The model under review builds one solid part; all positions refer to its coordinate system, in mm. Coordinates: 2 decimals unless noted, no trailing zeros. Write each loop counter-clockwise with the first axis right and the second up, starting at its lowest first coordinate (ties: lowest second). Pieces come first, ordered by that corner, then holes. Notation, with made-up numbers: (81.25, 13) - (128.25, 13) arc R34 cw to (128.25, 49) - close; hole circle Ø1 at (63.5, -38). An arc over 180 degrees is marked (long way). Put each result on its own line as item: value. Start each with the question number.
Item 1: For pin 1 (4.5 mm diameter, centred on x = 15.5, z = 50, fed in from -Y), flat-tipped, find the tip position at first contact; note if it passes through.
Item 2: Consider section A-A on x = -4.5. Give the boundary of the cut face in (y, z), then the cut area to 3 significant figures.
Item 3: To check wall thickness, follow L1, parallel to Z at x = 12.5, y = -35.15; L2, parallel to X at y = -33.75, z = 70; L3, parallel to Z at x = -14.5, y = -34.25. State the ranges of each line that lie inside material, in increasing order. Write a range as [from, to].
Item 4: Consider section D-D on x = 12.5. Give the boundary of the cut face in (y, z).
Item 5: Consider section C-C on z = 70. Give the boundary of the cut face in (x, y), then the cut area to 3 significant figures.
Item 6: Consider section B-B on z = 4.5. Give the boundary of the cut face in (x, y), then the cut area to 3 significant figures.
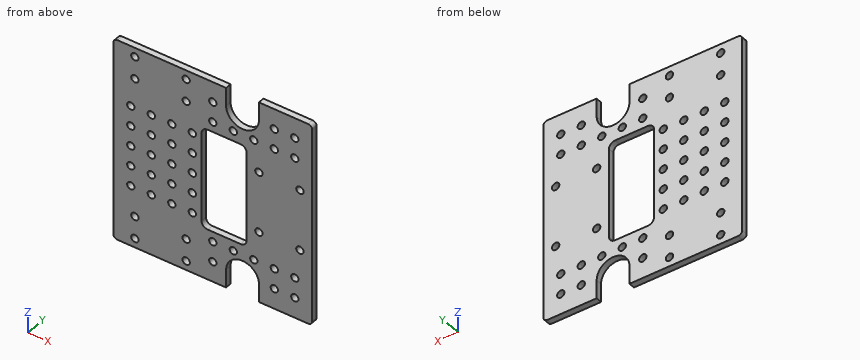
```python
from build123d import *

# Parameters (mm, degrees)
CYLINDER038_R            = 1.8
CYLINDER038_DEPTH        = 100
ARRAY001_X_COUNT         = 2
ARRAY001_X_PITCH         = 25
ARRAY001_Y_COUNT         = 2
ARRAY001_Y_PITCH         = 11
ARRAY001_PLACEMENT_ANGLE = 90
ARRAY002_Z_COUNT         = 2
ARRAY002_Z_PITCH         = 80
CYLINDER011003_R         = 1.8
CYLINDER011003_DEPTH     = 10
ARRAY005_X_COUNT         = 2
ARRAY005_X_PITCH         = 30
ARRAY005_Y_COUNT         = 2
ARRAY005_Y_PITCH         = 20
ARRAY005_PITCH_ANGLE     = 90
ARRAY005_PLACEMENT_ANGLE = -90
BOX002_W                 = 22
BOX002_H                 = 10
BOX002_DEPTH             = 50
FILLET002_R              = 3
BOX003_W                 = 16
BOX003_H                 = 200
BOX003_DEPTH             = 50
CYLINDER_R               = 8
CYLINDER_DEPTH           = 200
SKETCH_W                 = 42.117567
SKETCH_H                 = 23.738708
SKETCH_W_2               = 40.471139
SKETCH_H_2               = 27.047569
SKETCH_W_3               = 29.381024
SKETCH_H_3               = 46.19655
EXTRUDE_DEPTH            = 50
CYLINDER011002_R         = 1.8
CYLINDER011002_DEPTH     = 100
ARRAY004_X_COUNT         = 9
ARRAY004_X_PITCH         = 10
ARRAY004_Z_COUNT         = 9
ARRAY004_Z_PITCH         = 10
BOX_W                    = 97
BOX_H                    = 3
BOX_DEPTH                = 100
FILLET_R                 = 2


with BuildPart() as bolt_hole_array_pair:
    # Cylinder038 → Cylinder038 (new body)
    with BuildSketch(Plane.XY.offset(-50)):
        Circle(CYLINDER038_R)
    extrude(amount=CYLINDER038_DEPTH)

    # Array001 X: bolt hole array pair ×2


with BuildPart() as bolt_hole_array_pair_1:
    add(bolt_hole_array_pair.part)
    with Locations(*[(i * ARRAY001_X_PITCH, 0, 0) for i in range(1, ARRAY001_X_COUNT)]):
        add(bolt_hole_array_pair.part)

    # Array001 Y: bolt hole array pair ×2


with BuildPart() as bolt_hole_array_pair_2:
    add(bolt_hole_array_pair_1.part)
    with Locations(*[(0, i * ARRAY001_Y_PITCH, 0) for i in range(1, ARRAY001_Y_COUNT)]):
        add(bolt_hole_array_pair_1.part)


with BuildPart() as bolt_hole_array_pair_3:
    # Array001 placement: moved
    add(bolt_hole_array_pair_2.part.moved(Location((-12.5, 0, 4.5))).rotate(Axis((-12.5, 0, 4.5), (1, 0, 0)), ARRAY001_PLACEMENT_ANGLE))

    # Array002 Z: bolt hole array pair ×2


with BuildPart() as bolt_hole_array_pair_4:
    add(bolt_hole_array_pair_3.part)
    with Locations(*[(0, 0, i * ARRAY002_Z_PITCH) for i in range(1, ARRAY002_Z_COUNT)]):
        add(bolt_hole_array_pair_3.part)


with BuildPart() as stepper_mount_hole_array:
    # Cylinder011003 → Cylinder011003 (new body)
    with BuildSketch(Plane.XY):
        Circle(CYLINDER011003_R)
    extrude(amount=CYLINDER011003_DEPTH)

    # Array005 X: stepper mount hole array ×2


with BuildPart() as stepper_mount_hole_array_1:
    add(stepper_mount_hole_array.part)
    with Locations(*[(i * ARRAY005_X_PITCH, 0, 0) for i in range(1, ARRAY005_X_COUNT)]):
        add(stepper_mount_hole_array.part)

    # Array005 Y: stepper mount hole array ×2


with BuildPart() as stepper_mount_hole_array_2:
    add(stepper_mount_hole_array_1.part)
    with Locations(*[(0, i * ARRAY005_Y_PITCH, 0) for i in range(1, ARRAY005_Y_COUNT)]):
        add(stepper_mount_hole_array_1.part)


with BuildPart() as stepper_mount_hole_array_3:
    # Array005 pitch: moved
    add(stepper_mount_hole_array_2.part.rotate(Axis((0, 0, 0), (0, 1, 0)), ARRAY005_PITCH_ANGLE))


with BuildPart() as stepper_mount_hole_array_4:
    # Array005 placement: moved
    add(stepper_mount_hole_array_3.part.moved(Location((48, -31, 65))).rotate(Axis((48, -31, 65), (0, 0, 1)), ARRAY005_PLACEMENT_ANGLE))


with BuildPart() as belt_hole_fillet:
    # Box002 → Box002 (new body)
    with BuildSketch(Plane(origin=(20, -40, 25), x_dir=(1, 0, 0), z_dir=(0, 0, 1))):
        with Locations((11, 5)):
            Rectangle(BOX002_W, BOX002_H)
    extrude(amount=BOX002_DEPTH)

    # Fillet002
    fillet002_edges = [belt_hole_fillet.edges().sort_by_distance(p)[0] for p in [
        (20, -35, 75),
        (20, -35, 25),
        (42, -35, 75),
        (42, -35, 25),
    ]]
    fillet(fillet002_edges, radius=FILLET002_R)


with BuildPart() as shaft_extension_cube:
    # Box003 → Box003 (new body)
    with BuildSketch(Plane(origin=(-8, -200, -50), x_dir=(1, 0, 0), z_dir=(0, 0, 1))):
        with Locations((8, 100)):
            Rectangle(BOX003_W, BOX003_H)
    extrude(amount=BOX003_DEPTH)


with BuildPart() as shaft_16mm_hole:
    # Cylinder → Cylinder (new body)
    with BuildSketch(Plane.XZ):
        Circle(CYLINDER_R)
    extrude(amount=CYLINDER_DEPTH)

    # Fusion002: union shaft extension cube
    add(shaft_extension_cube.part)


with BuildPart() as shaft_16mm_hole_1:
    # Fusion002 placement: moved
    add(shaft_16mm_hole.part.moved(Location((40, -19, 9))))


with BuildPart() as part_mirroring:
    # Part__Mirroring: instance of shaft 16mm hole
    add(shaft_16mm_hole_1.part.mirror(Plane(origin=(0, 0, 50), x_dir=(0, 1, 0), z_dir=(0, 0, 1))))


with BuildPart() as general_holes_extrude:
    # Sketch → Extrude (new body, symmetric)
    with BuildSketch(Plane.XZ):
        with Locations((-1.795196, 11.674214)):
            Rectangle(SKETCH_W, SKETCH_H)
        with Locations((-0.985158, 89.151065)):
            Rectangle(SKETCH_W_2, SKETCH_H_2)
        with Locations((57.017252, 49.302802)):
            Rectangle(SKETCH_W_3, SKETCH_H_3)
    extrude(amount=EXTRUDE_DEPTH, both=True)


with BuildPart() as hole_fusion:
    # Cylinder011002 → Cylinder011002 (new body)
    with BuildSketch(Plane.XZ.offset(-50)):
        Circle(CYLINDER011002_R)
    extrude(amount=CYLINDER011002_DEPTH)

    # Array004 X: hole fusion ×9


with BuildPart() as hole_fusion_1:
    add(hole_fusion.part)
    with Locations(*[(i * ARRAY004_X_PITCH, 0, 0) for i in range(1, ARRAY004_X_COUNT)]):
        add(hole_fusion.part)

    # Array004 Z: hole fusion ×9


with BuildPart() as hole_fusion_2:
    add(hole_fusion_1.part)
    with Locations(*[(0, 0, i * ARRAY004_Z_PITCH) for i in range(1, ARRAY004_Z_COUNT)]):
        add(hole_fusion_1.part)


with BuildPart() as hole_fusion_3:
    # Array004 placement: moved
    add(hole_fusion_2.part.moved(Location((-14.5, 0, 10))))

    # Cut: cut general holes extrude
    add(general_holes_extrude.part, mode=Mode.SUBTRACT)

    # Fusion: union bolt hole array pair, stepper mount hole array, belt hole fillet, Part__Mirroring, shaft 16mm hole
    add(bolt_hole_array_pair_4.part)
    add(stepper_mount_hole_array_4.part)
    add(belt_hole_fillet.part)
    add(part_mirroring.part)
    add(shaft_16mm_hole_1.part)


with BuildPart() as side_plate_cut:
    # Box → Box (new body)
    with BuildSketch(Plane(origin=(-23, -36, 0), x_dir=(1, 0, 0), z_dir=(0, 0, 1))):
        with Locations((48.5, 1.5)):
            Rectangle(BOX_W, BOX_H)
    extrude(amount=BOX_DEPTH)

    # Fillet
    fillet_edges = [side_plate_cut.edges().sort_by_distance(p)[0] for p in [
        (-23, -34.5, 100),
        (-23, -34.5, 0),
        (74, -34.5, 100),
        (74, -34.5, 0),
    ]]
    fillet(fillet_edges, radius=FILLET_R)

    # Cut023015009002: cut hole fusion
    add(hole_fusion_3.part, mode=Mode.SUBTRACT)


solid = side_plate_cut.part
```
Report:
1. pin 1: y = -36
2. outline: (-36, 0) - (-33, 0) - (-33, 28.2) - (-36, 28.2) - close; (-36, 31.8) - (-33, 31.8) - (-33, 38.2) - (-36, 38.2) - close; (-36, 41.8) - (-33, 41.8) - (-33, 48.2) - (-36, 48.2) - close; (-36, 51.8) - (-33, 51.8) - (-33, 58.2) - (-36, 58.2) - close; (-36, 61.8) - (-33, 61.8) - (-33, 68.2) - (-36, 68.2) - close; (-36, 71.8) - (-33, 71.8) - (-33, 100) - (-36, 100) - close
2. area: 246 mm²
3. L1: [0, 2.7], [6.3, 13.7], [17.3, 82.7], [86.3, 93.7], [97.3, 100]
3. L2: [-23, -16.3], [-12.7, -6.3], [-2.7, 3.7], [7.3, 13.7], [17.3, 20], [42, 74]
3. L3: [0, 28.2], [31.8, 38.2], [41.8, 48.2], [51.8, 58.2], [61.8, 68.2], [71.8, 100]
4. outline: (-36, 0) - (-33, 0) - (-33, 2.7) - (-36, 2.7) - close; (-36, 6.3) - (-33, 6.3) - (-33, 13.7) - (-36, 13.7) - close; (-36, 17.3) - (-33, 17.3) - (-33, 82.7) - (-36, 82.7) - close; (-36, 86.3) - (-33, 86.3) - (-33, 93.7) - (-36, 93.7) - close; (-36, 97.3) - (-33, 97.3) - (-33, 100) - (-36, 100) - close
5. outline: (-23, -36) - (-16.3, -36) - (-16.3, -33) - (-23, -33) - close; (-12.7, -36) - (-6.3, -36) - (-6.3, -33) - (-12.7, -33) - close; (-2.7, -36) - (3.7, -36) - (3.7, -33) - (-2.7, -33) - close; (7.3, -36) - (13.7, -36) - (13.7, -33) - (7.3, -33) - close; (17.3, -36) - (20, -36) - (20, -33) - (17.3, -33) - close; (42, -36) - (74, -36) - (74, -33) - (42, -33) - close
5. area: 182 mm²
6. outline: (-23, -36) - (-14.3, -36) - (-14.3, -33) - (-23, -33) - close; (-10.7, -36) - (10.7, -36) - (10.7, -33) - (-10.7, -33) - close; (14.3, -36) - (32, -36) - (32, -33) - (14.3, -33) - close; (48, -36) - (74, -36) - (74, -33) - (48, -33) - close
6. area: 221 mm²
